The figure shows three views and two pictorial views of one solid part (mm, origin at its lowest corner). Answer the questions. A direction names the side the tool comes from. Give positions to 0.01 mm unless a question says otherwise; leave off trailing zeros. Loops run counter-clockwise (first coordinate to the right, second up) from the corner with the lowest first, then second, coordinate; pieces in that order, holes last. Notation, with made-up numbers: M -37.75,43 L 15.25,43 A16 cw 15.25,66 Z; hole C -8.75,63.5 d5. An arc over 180 degrees is marked long. Answer as a JSON object with one key per item and string values. Group by question number.
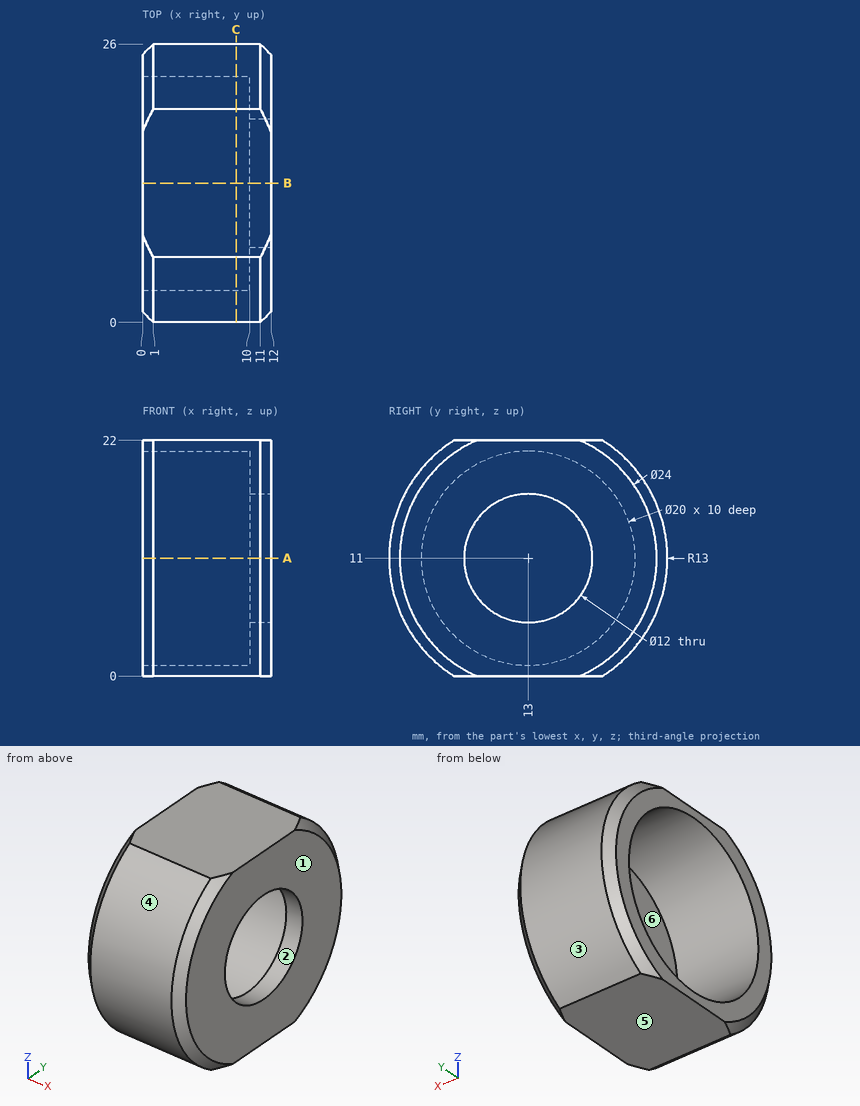
Item 1: Find the intervals of material crossed by probe 1 along Z at (x, y) = (11.4, 13); probe 2 along Z at (x, y) = (5.5, 13); probe 3 along X at (y, z) = (6.75, 4), in increasing order. Write a range as [from, to].
Item 2: A cutting plane is placed at C-C (x = 8.75). Determine the outline of the cut face in (y, z).
Item 3: A cutting plane is placed at B-B (y = 13). Determine the outline of the cut face in (x, z), and give its area (3 significant figures).
Item 4: A tool of negligible diameter and unlimited length cuts with its end or side. For the marked faces 5 and 6, from which of +Z, -Z, +X, -X, +Y, -Y can it reach the whole face along a straight path? Write none if from no direction.
Item 5: For a pull along Y with two mould halves and no side action, classify the marked faces 1, 2, 3 and 4 as pulls with the +Y half, pulls with the -Y half, needs draft (parallel to the pull), parting line crosses it, or undercut.
Item 6: A cutting plane is placed at A-A (z = 11). Determine the outline of the cut face in (x, y).
Item 7: Given pin 1 Ø3 at (x, y) = (5, 5.5) entering from +Z; pin 2 Ø1.5 at (y, z) = (10, 17.5) entering from -X; pin 3 Ø1.5 at (x, z) = (10, 15.5) entering from +Y; pin 4 Ø1.5 at (x, z) = (1.5, 15) entering from +Y, each flat-ended and moving along its own axis, determine where each tip first touches the part or whether it passes through.
The answers:
{
 "1": {"probe 1": "z = [0, 5], [17, 22]", "probe 2": "z = [0, 1], [21, 22]", "probe 3": "x = [10, 12]"},
 "2": {"outline": "M 6.07,0 L 19.93,0 A13 ccw 19.93,22 L 6.07,22 A13 ccw Z; hole C 13,11 d20"},
 "3": {"outline": "M 0,0 L 12,0 L 12,5 L 10,5 L 10,1 L 0,1 Z; M 0,21 L 10,21 L 10,17 L 12,17 L 12,22 L 0,22 Z", "area": "40.0 mm^2"},
 "4": {"face 5": "-Z, +X, -X, +Y, -Y", "face 6": "-X"},
 "5": {"face 1": "needs draft", "face 2": "undercut", "face 3": "pulls with the +Y half", "face 4": "pulls with the -Y half"},
 "6": {"outline": "M 0,1 L 1,0 L 11,0 L 12,1 L 12,7 L 10,7 L 10,3 L 0,3 Z; M 0,23 L 10,23 L 10,19 L 12,19 L 12,25 L 11,26 L 1,26 L 0,25 Z"},
 "7": {"pin 1": "stops at z = 22", "pin 2": "stops at x = 10", "pin 3": "stops at y = 25.45", "pin 4": "stops at y = 25.59"}
}
